Work out the finished part from the listing and answer in its coordinate system (mm). Face numbers are marked on the shaded views. A direction names the side the tool comes from. Round coordinates to 2 decimals unless told otherwise and drop trailing zeros. Write each loop counter-clockwise with the first axis right and the second up, starting at its lowest first coordinate (ties: lowest second). Pieces come first, ordered by that corner, then holes. Notation, with made-up numbers: (-39.5, 32.25) -> (-33.5, 32.25) arc R19 ccw to (-33.5, 54.25) -> close; hole circle Ø5 at (20.5, 25). An arc over 180 degrees is marked (long way). One line per item, written item: value.
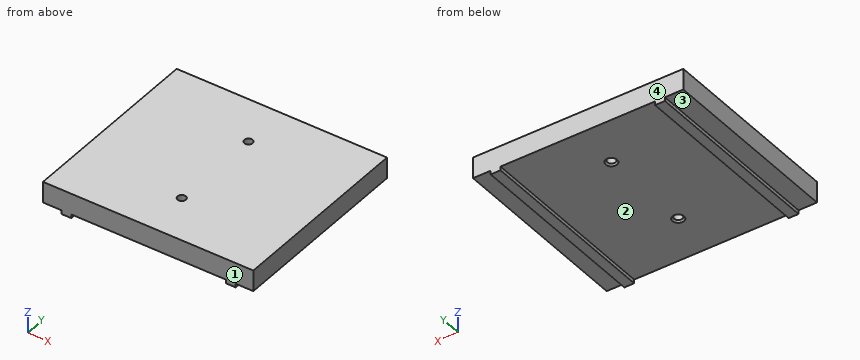
Autodesk Inventor part; units mm, degrees
ref_plane "YZ Plane" through (0, 0, 0) normal (1, 0, 0) x (0, 1, 0)
ref_plane "XZ Plane" through (0, 0, 0) normal (0, 1, 0) x (-1, 0, 0)
ref_plane "XY Plane" through (0, 0, 0) normal (0, 0, 1) x (1, 0, 0)
sketch "Sketch1" plane through (0, 0, 0) normal (0, 0, 1) x (1, 0, 0)
  line L0 (86.5564, -16.51) -> (86.5564, 16.51)
  line L1 (93.1064, -19.05) -> (93.1064, 19.05)
  line L2 (86.5564, 19.05) -> (86.5564, -19.05)
  line L3 (93.1064, -19.05) -> (93.1064, 19.05)
  line L4 (-12.6968, 19.05) -> (-12.6968, -19.05)
  line L5 (-6.1468, -19.05) -> (-6.1468, 19.05)
  line L6 (-12.6968, -31.75) -> (-12.6968, -69.85)
  line L7 (-6.1468, -69.85) -> (-6.1468, -31.75)
  line L8 (86.5564, -31.75) -> (86.5564, -69.85)
  line L9 (93.1064, -69.85) -> (93.1064, -31.75)
  line L10 (-12.6968, -19.05) -> (-12.6968, -31.75)
  line L11 (-6.1468, -31.75) -> (-6.1468, -19.05)
  line L12 (-12.3968, -19.05) -> (-12.3968, 18.85)
  line L13 (-6.4516, 18.85) -> (-6.4516, -19.05)
  line L14 (-6.4516, -19.05) -> (-6.4516, -31.75)
  line L15 (-6.4516, -31.75) -> (-6.4516, -69.65)
  line L16 (-12.3968, -69.65) -> (-12.3968, -31.75)
  line L17 (-12.3968, -31.75) -> (-12.3968, -19.05)
  line L18 (8.247, -25.4) -> (71.6799, -25.4) construction
  line L19 (39.9635, 46.4598) -> (39.9635, -93.3096) construction
  line L20 (-23.5365, 31.75) -> (103.4635, 31.75)
  line L21 (103.4635, 31.75) -> (103.4635, -82.55)
  line L22 (103.4635, -82.55) -> (-23.5365, -82.55)
  line L23 (-23.5365, -82.55) -> (-23.5365, 31.75)
  line L24 (-23.5365, 31.75) -> (103.4635, -82.55) construction
  line L25 (103.4635, 31.75) -> (-23.5365, -82.55) construction
  line L26 (86.5564, -19.05) -> (86.5564, -31.75)
  line L27 (93.1064, -31.75) -> (93.1064, -19.05)
  line L28 (86.5564, 19.05) -> (86.5564, 31.75)
  line L29 (93.1064, 19.05) -> (93.1064, 31.75)
  line L30 (93.1064, -69.85) -> (93.1064, -82.55)
  line L31 (86.5564, -69.85) -> (86.5564, -82.55)
  line L32 (-12.3968, 18.85) -> (-12.3968, 31.75)
  line L33 (-6.4516, 18.85) -> (-6.4516, 31.75)
  line L34 (-6.1468, -69.85) -> (-6.1468, -82.55)
  line L35 (-12.3968, -69.65) -> (-12.3968, -82.55)
  line L36 (-12.6968, 19.05) -> (-12.6968, 31.75)
  line L37 (-6.1468, 19.05) -> (-6.1468, 31.75)
  line L38 (-12.6968, -69.85) -> (-12.6968, -82.55)
  line L39 (-6.4516, -69.65) -> (-6.4516, -82.55)
  line L40 (86.8564, 31.75) -> (86.8564, 19.05)
  line L41 (86.8564, 19.05) -> (86.8564, -19.05)
  line L42 (86.8564, -19.05) -> (86.8564, -31.75)
  line L43 (86.8564, -31.75) -> (86.8564, -69.85)
  line L44 (86.8564, -69.85) -> (86.8564, -82.55)
  line L45 (93.1064, 31.75) -> (93.1064, -82.55)
  line L46 (93.1064, 31.75) -> (93.1064, -82.55)
  line L47 (92.8064, 31.75) -> (92.8064, -82.55)
  point P0 (0, 0)
  point P1 (93.1064, -16.51)
  point P2 (39.9635, -25.4)
  dimension "d0" = 0.3
  dimension "d1" = 127
  dimension "d2" = 114.3
  dimension "d7" = 0.3
  dimension "d8" = 0.3
  dimension "d9" = 0.3048
extrude "Extrusion1" add sketch "Sketch1" against normal blind 2.286 contours L20 L47 L22 L44 L43 L42 L41 L40 | L33 L13 L14 L15 L39 L22 L35 L16 L17 L12 L32 L20
sketch "Sketch2" plane through (0, 0, 0) normal (0, 0, 1) x (1, 0, 0)
  line L0 (103.4635, 31.75) -> (103.4635, -82.55)
  line L1 (-23.5365, 31.75) -> (103.4635, 31.75)
  line L2 (-23.5365, -82.55) -> (-23.5365, 31.75)
  line L3 (103.4635, -82.55) -> (-23.5365, -82.55)
  point P0 (0, 0)
  point P1 (93.1064, 31.75)
extrude "Extrusion2" add sketch "Sketch2" along normal blind 12.7
sketch "Sketch3" plane through (0, 0, 12.7) normal (0, 0, 1) x (1, 0, 0)
  line L0 (-23.5365, 31.75) -> (-23.5365, -82.55)
  line L1 (-23.5365, -82.55) -> (103.4635, -82.55)
  line L2 (103.4635, -82.55) -> (103.4635, 31.75)
  line L3 (103.4635, 31.75) -> (-23.5365, 31.75)
  point P0 (0, 0)
sketch "Sketch4" plane through (0, 0, 0) normal (0, 0, -1) x (-1, 0, 0)
  line L0 (6.4516, -82.55) -> (6.4516, 31.75)
  line L1 (-86.8564, 31.75) -> (6.4516, 31.75)
  line L2 (-86.8564, 31.75) -> (-86.8564, -82.55)
  line L3 (6.4516, -82.55) -> (-86.8564, -82.55)
  line L4 (-39.9406, -25.4) -> (-40.2024, 31.75) construction
  circle A0 centre (-40.0715, 3.175) radius 2.5
  line L5 (-8.2452, -25.4007) -> (-71.9453, -25.4007) construction
  circle A1 centre (-40.0715, -53.9764) radius 2.5
  point P0 (0, 0)
  dimension "d10" = 5
extrude "Extrusion3" cut sketch "Sketch4" against normal up to surface (12.7 mm away) contours A0 | A1
chamfer "Chamfer1" distance 1 angle 45 2 edges at (42.5715, 3.175, 0) (42.5715, -53.9764, 0)
properties part number "CartTrack"
(1) Flat-ended cylindrical pins translate along their axes: pin 1 Ø0.7 at (y, z) = (-38, -1.5) entering from -X; pin 2 Ø1.8 at (y, z) = (-22.5, -1) entering from +X; pin 3 Ø6.5 at (x, y) = (40.07, -53.98) entering from -Z. Find the tip coordinate at first contact, or state that the pin passes through.
Reported:
pin 1: stops at x = -12.4
pin 2: stops at x = 92.81
pin 3: stops at z = 0.25
(2) A tool of negligible diameter and unlimited length cuts with its end or side. For the marked faces 3 and 4, from which of +Z, -Z, +X, -X, +Y, -Y can it reach the whole face along a straight path? Write none if from no direction.
Reported:
face 3: -Z, -X, +Y, -Y
face 4: +Z, -Z, +X, -X, +Y
(3) Find section B-B on x = 25. Give the vertices of the cut face in (y, z).
Reported:
outline: (-82.55, 0) -> (31.75, 0) -> (31.75, 12.7) -> (-82.55, 12.7) -> close
(4) For a pull along X with two mould halves and no side action, classify the marked faces 1 and 2 as pulls with the +X half, pulls with the -X half, needs draft (parallel to the pull), parting line crosses it, or undercut.
Reported:
face 1: needs draft
face 2: undercut
(5) Consider probe 1 along X at (y, z) = (12, -0.75); probe 2 along X at (y, z) = (-54, 6); probe 3 along Z at (x, y) = (66.5, -70). Determine where each line is inside the solid, lowest interval first.
Reported:
probe 1: x = -12.4 to -6.45, 86.86 to 92.81
probe 2: x = -23.54 to 37.57, 42.57 to 103.46
probe 3: z = 0 to 12.7
(6) Find section A-A on y = -47. Give the vertices of the cut face in (x, z).
Reported:
outline: (-23.54, 0) -> (-12.4, 0) -> (-12.4, -2.29) -> (-6.45, -2.29) -> (-6.45, 0) -> (86.86, 0) -> (86.86, -2.29) -> (92.81, -2.29) -> (92.81, 0) -> (103.46, 0) -> (103.46, 12.7) -> (-23.54, 12.7) -> close
